Geometry: see drawing. Coordinates: mm, zero at the bounding-box minimum. Coordinates: 2 decimals unless noted, no trailing zeros. Use a Markdown table: item, result. Add a question column.
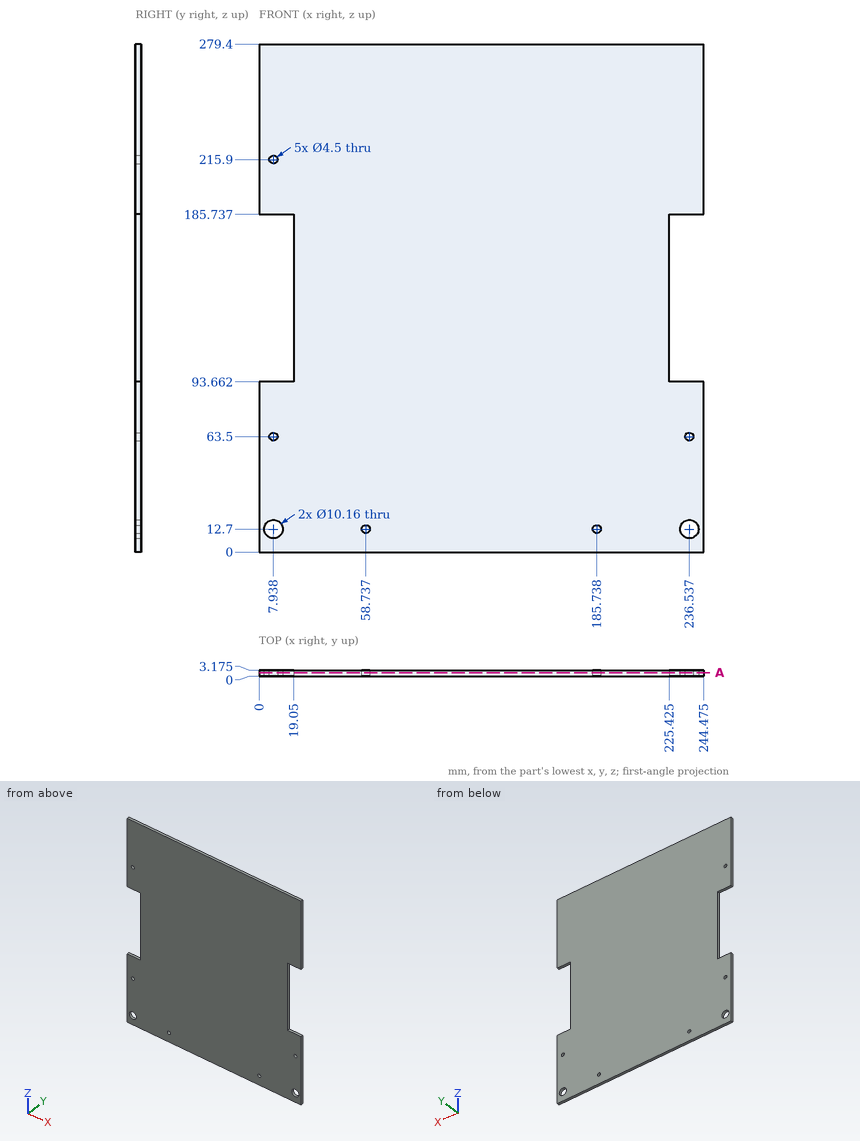
1) First-contact query: pin 1 (8 mm diameter, centred on x = 7.94, z = 12.7, fed in from +Y) (3 decimals); pin 2 (1 mm diameter, centred on y = 2.5, z = 117.5, fed in from -X). Flat tips, straight axial feed; report the tip coordinate or a pass-through.
2) Line query: line 1 (X direction, y = 1.05, z = 63.5) (1 decimal); line 2 (X direction, y = 1.55, z = 12.7) (1 decimal); line 3 (Z direction, x = 227, y = 2.35). Output: solid intervals per line, ascending. Write a range as from..to.
3) Section query A-A (y = 1.8). Give the number of separate pieces and of enclosed holes in the cut face, and give its area (3 significant figures).
From the geometry:
| question | item | result |
|---|---|---|
| 1 | pin 1 | passes through |
| 1 | pin 2 | stops at x = 19.05 |
| 2 | line 1 | x = 0..5.7, 10.2..234.3, 238.8..244.5 |
| 2 | line 2 | x = 0..2.9, 13..56.5, 61..183.5, 188..231.5, 241.6..244.5 |
| 2 | line 3 | z = 0..93.66, 185.74..279.4 |
| 3 | separate pieces | 1 |
| 3 | enclosed holes | 7 |
| 3 | area | 64,600 mm^2 |
